Study the drawing (mm; zero at the part's minimum x, y, z) and answer. A direction names the side the tool comes from. Round coordinates to 2 decimals unless told otherwise and drop trailing zeros. Order: outer loops, then holes, each group sorted by start corner. A loop starts at its lowest first (then second) coordinate and runs counter-clockwise, first axis right, second up. Notation, with made-up numbers: M 57,-27 L 116,-27 A10 cw 116,-14 Z; hole C 15,-2 d2. An arc over 180 degrees is marked long. Put each result on its own line as item: value. Start each with the question number.
1. Consider line 1 (Y direction, x = 79, z = 10) (1 decimal); line 2 (X direction, y = 10, z = 32); line 3 (Z direction, x = 77, y = 15). Determine where each line is inside the solid, lowest interval first.
2. The mould has two halves that part along Y. Classify the marked faces 4, 5, 6 and 7: +Y half, -Y half, draft (parallel to the pull), parting line (faces both ways), or undercut.
3. The part is cut by section B-B (z = 34.5). Give the vertices of the cut face in (x, y) (1 decimal), then the cut area to 3 significant figures.
4. Each of these flat-tipped pins is pushed along its axis until it touches: pin 1 Ø1.5 at (x, y) = (85.5, 47.5) entering from +Z; pin 2 Ø15 at (x, z) = (104, 11) entering from -Y; pin 3 Ø12.5 at (x, y) = (13, 35.5) entering from +Z. Where does it stop, or does it pass through?
5. Which of the six approach directions +Z, -Z, +X, -X, +Y, -Y give full straight-line access (tool end or side, diameter ignored) to the marked faces 1, 2 and 3?
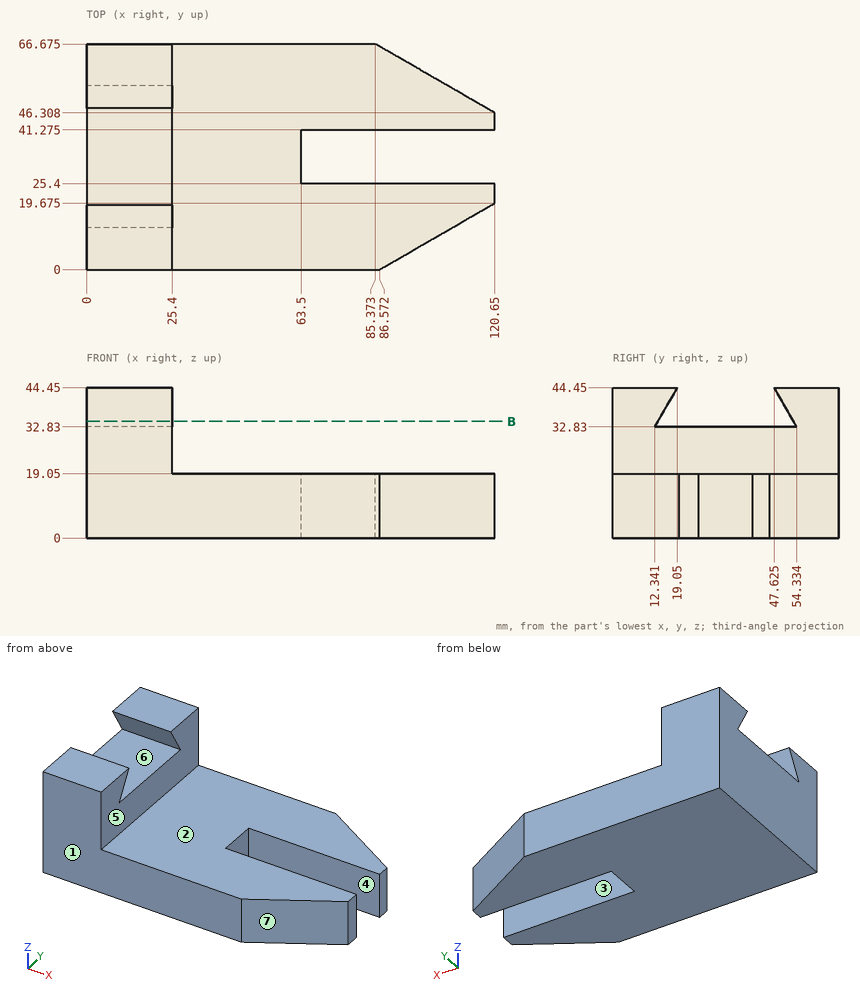
Resolved:
1. line 1: 0 to 25.4, 41.3 to 66.7
1. line 2: 0 to 25.4
1. line 3: 0 to 19.05
2. face 4: undercut
2. face 5: draft
2. face 6: undercut
2. face 7: -Y half
3. outline: M 0,0 L 25.4,0 L 25.4,13.3 L 0,13.3 Z; M 0,53.4 L 25.4,53.4 L 25.4,66.7 L 0,66.7 Z
3. area: 676 mm2
4. pin 1: z = 19.05
4. pin 2: y = 5.73
4. pin 3: z = 32.83
5. face 1: +Z, -Z, +X, -X, -Y
5. face 2: +Z, +X, +Y, -Y
5. face 3: +Z, -Z, +X
